```python
from build123d import *

# Parameters (mm, degrees)
SKETCH2_R                   = 8.255
BOSS_EXTRUDE1_DEPTH         = 6.35
BOSS_EXTRUDE1_DEPTH_BACK    = 6.35
BOSS_EXTRUDE2_DEPTH         = 10.16
BOSS_EXTRUDE2_DEPTH_BACK    = 16.256
SKETCH4_W                   = 20.32
SKETCH4_H                   = 10.16
BOSS_EXTRUDE3_DEPTH         = 10.16
BOSS_EXTRUDE3_DEPTH_BACK    = 16.51
SKETCH5_W                   = 20.32
SKETCH5_H                   = 10.16
CUT_EXTRUDE1_DEPTH          = 372.505050517
CUT_EXTRUDE2_DEPTH          = 370.547039673
CUT_EXTRUDE3_START          = -16.256
CUT_EXTRUDE3_DEPTH          = 16.256
CUT_EXTRUDE4_DEPTH          = 16.51
E_0_25_DIAMETER_HOLE1_D     = 6.35
E_0_25_DIAMETER_HOLE1_DEPTH = 19.05
E_0_25_DIAMETER_HOLE1_TIP   = 1.907732465
CUT_EXTRUDE5_DEPTH          = 367.61301524
CUT_EXTRUDE5_DEPTH_BACK     = 367.61301524
SKETCH13_R                  = 3.175


with BuildPart() as part:
    # Sweep1: sweep along a path in Sketch1
    with BuildLine(Plane(origin=(0, 0, 0), x_dir=(1, 0, 0), z_dir=(0, 1, 0))) as sweep1_path:
        Line((-307.263447944, -157.854259231), (0, 0))
        Line((0, 0), (-307.263447944, 172.345740769))
    # Sketch2 → Sweep1 (sweep)
    with BuildSketch(Plane(origin=(-307.263447944, 0, 157.854259231), x_dir=(-0.45696578054298637, 0, -0.8894842749665333), z_dir=(0.8894842749665333, 0, -0.45696578054298637))):
        Circle(SKETCH2_R)
    sweep(path=sweep1_path.line, transition=Transition.RIGHT)

    # Sketch3 → Boss-Extrude1 (add, two sides: drawn at the far end of the back side and taken through both)
    with BuildSketch(Plane.XY.offset(-BOSS_EXTRUDE1_DEPTH_BACK)):
        Polygon((33.931753368, 10.795), (11.09345, 10.795), (11.09345, -10.795), (33.931753368, -10.795), (33.931753368, -7.62), (14.26845, -7.62), (14.26845, 7.62), (33.931753368, 7.62), align=None)
    extrude(amount=BOSS_EXTRUDE1_DEPTH + BOSS_EXTRUDE1_DEPTH_BACK)

    # Sketch4 → Boss-Extrude2 (add, two sides: drawn at the far end of the back side and taken through both)
    with BuildSketch(Plane(origin=(-307.263447944, 0, 157.854259231), x_dir=(0.45696578054298637, 0, 0.8894842749665333), z_dir=(-0.8894842749665333, 0, 0.45696578054298637)).offset(-BOSS_EXTRUDE2_DEPTH_BACK)):
        Rectangle(SKETCH4_W, SKETCH4_H)
    extrude(amount=BOSS_EXTRUDE2_DEPTH + BOSS_EXTRUDE2_DEPTH_BACK)

    # Sketch5 → Boss-Extrude3 (add, two sides: drawn at the far end of the back side and taken through both)
    with BuildSketch(Plane(origin=(-307.263447944, 0, -172.345740769), x_dir=(-0.4892044257112748, 0, 0.8721691520940774), z_dir=(-0.8721691520940774, 0, -0.4892044257112748)).offset(-BOSS_EXTRUDE3_DEPTH_BACK)):
        Rectangle(SKETCH5_W, SKETCH5_H)
    extrude(amount=BOSS_EXTRUDE3_DEPTH + BOSS_EXTRUDE3_DEPTH_BACK)

    # Sketch6 → Cut-Extrude1 (cut, through all)
    with BuildSketch(Plane(origin=(0, 5.08, 0), x_dir=(1, 0, 0), z_dir=(0, 1, 0))):
        with BuildLine():
            Line((-312.23376491, 163.484502184), (-321.095003495, 168.454819149))
            Line((-321.095003495, 168.454819149), (-316.12468653, 177.316057734))
            ThreePointArc((-316.12468653, 177.316057734), (-317.043834669, 169.594443707), (-312.23376491, 163.484502184))
        make_face()
    cut_extrude1 = extrude(amount=-CUT_EXTRUDE1_DEPTH, mode=Mode.SUBTRACT)

    # Mirror1: Cut-Extrude1 across plane
    add(cut_extrude1.mirror(Plane(origin=(0, 0, 0), x_dir=(0.8721691520940776, 0, 0.48920442571127426), z_dir=(-0.4892044257112748, 0, 0.8721691520940775))), mode=Mode.SUBTRACT)

    # Sketch7 → Cut-Extrude2 (cut, through all)
    with BuildSketch(Plane(origin=(0, 5.08, 0), x_dir=(1, 0, 0), z_dir=(0, 1, 0))):
        with BuildLine():
            Line((-302.620675614, -166.891419464), (-311.657835848, -171.534191795))
            Line((-311.657835848, -171.534191795), (-316.300608178, -162.497031561))
            ThreePointArc((-316.300608178, -162.497031561), (-310.37074943, -167.527432313), (-302.620675614, -166.891419464))
        make_face()
    cut_extrude2 = extrude(amount=-CUT_EXTRUDE2_DEPTH, mode=Mode.SUBTRACT)

    # Mirror2: Cut-Extrude2 across plane
    add(cut_extrude2.mirror(Plane(origin=(0, 0, 0), x_dir=(-0.8894842749665333, 0, 0.45696578054298614), z_dir=(0.45696578054298637, 0, 0.8894842749665333))), mode=Mode.SUBTRACT)

    # Sketch8 → Cut-Extrude3 (cut)
    with BuildSketch(Plane(origin=(-307.263447944, 0, 157.854259231), x_dir=(0.45696578054298637, 0, 0.8894842749665333), z_dir=(-0.8894842749665333, 0, 0.45696578054298637)).offset(CUT_EXTRUDE3_START)):
        with BuildLine():
            Line((6.506813736, -5.08), (-6.506813736, -5.08))
            ThreePointArc((-6.506813736, -5.08), (0, -8.255), (6.506813736, -5.08))
        make_face()
        with BuildLine():
            Line((-6.506813736, 5.08), (6.506813736, 5.08))
            ThreePointArc((6.506813736, 5.08), (0, 8.255), (-6.506813736, 5.08))
        make_face()
    extrude(amount=CUT_EXTRUDE3_DEPTH, mode=Mode.SUBTRACT)

    # Sketch9 → Cut-Extrude4 (cut)
    with BuildSketch(Plane(origin=(-307.263447944, 0, -172.345740769), x_dir=(-0.4892044257112748, 0, 0.8721691520940774), z_dir=(-0.8721691520940774, 0, -0.4892044257112748))):
        with BuildLine():
            Line((6.506813736, -5.08), (-6.506813736, -5.08))
            ThreePointArc((-6.506813736, -5.08), (0, -8.255), (6.506813736, -5.08))
        make_face()
        with BuildLine():
            Line((-6.506813736, 5.08), (6.506813736, 5.08))
            ThreePointArc((6.506813736, 5.08), (0, 8.255), (-6.506813736, 5.08))
        make_face()
    extrude(amount=-CUT_EXTRUDE4_DEPTH, mode=Mode.SUBTRACT)

    # E (0.25) Diameter Hole1
    with Locations(Plane(origin=(-307.263447944, 5.08, -172.345740769), x_dir=(0, 0, 1), z_dir=(0, 1, 0))):
        with Locations((0, 0), (330.2, 0)):
            Hole(E_0_25_DIAMETER_HOLE1_D / 2, depth=E_0_25_DIAMETER_HOLE1_DEPTH)
            with Locations((0, 0, -(E_0_25_DIAMETER_HOLE1_DEPTH + E_0_25_DIAMETER_HOLE1_TIP / 2))):  # 118° drill point
                Cone(0, E_0_25_DIAMETER_HOLE1_D / 2, E_0_25_DIAMETER_HOLE1_TIP, mode=Mode.SUBTRACT)

    # Sketch13 → Cut-Extrude5 (cut, two sides: drawn at the far end of the back side and taken through both)
    with BuildSketch(Plane(origin=(0, -7.62, 0), x_dir=(1, 0, 0), z_dir=(0, 1, 0)).offset(-CUT_EXTRUDE5_DEPTH_BACK)):
        with Locations(Location((24.100101684, 0, 0), (0, 0, 180))):
            Circle(SKETCH13_R)
    extrude(amount=CUT_EXTRUDE5_DEPTH + CUT_EXTRUDE5_DEPTH_BACK, mode=Mode.SUBTRACT)


solid = part.part
```
The listing builds one solid part. Answer for the finished solid, in the listing's coordinates (mm). A direction names the side the tool comes from. Give positions to 0.01 mm unless a question says otherwise; leave off trailing zeros. One line per item, written item: value.
1) Flat-ended cylindrical pins translate along their axes: P1, Ø1.5, axis at y = 2, z = -36, coming from the +X side; P2, Ø4, axis at y = -3.5, z = 1.5, coming from the -X side; P3, Ø1.5, axis at y = 1, z = 22, coming from the -X side; P4, Ø10, axis at x = 22, z = 0, coming from the +Y side (3 decimals). Find the tip coordinate at first contact, or state that the pin passes through.
Reported:
P1: stops at x = -46.42
P2: stops at x = -23.56
P3: stops at x = -62.23
P4: stops at y = 10.795
2) A tool of negligible diameter and unlimited length cuts with its end or side. For faces 4 (the flat face through (-304, 5.08, -171)), 5 (the flat face through (14.268, 0, -2)), 6 (the flat face through (14, 0, 6.35)), 7 (the flat face through (-304.575, -0.071, 145.051)), 8 (the flat face through (-304, 5.08, 156)), from which of +Z, -Z, +X, -X, +Y, -Y can it reach the whole face along a straight path? Write none if from no direction.
Reported:
face 4: -Z, -X, +Y
face 5: +X
face 6: +Z, +X, +Y, -Y
face 7: -X, +Y, -Y
face 8: +Z, -X, +Y
3) Determine the mould class of faces 1 (the flat face through (11.093, 3, -3)), 2 (the flat face through (-304, -5.08, 156)), 3 (the flat face through (-304.93, -0.07, -159.39)) for opening direction X: pulls with the +X half, pulls with the -X half, needs draft (parallel to the pull), parting line crosses it, or undercut.
Reported:
face 1: undercut
face 2: needs draft
face 3: pulls with the -X half
4) Find the intervals of material crossed by line 1 (X direction, y = -9.5, z = 0); line 2 (Z direction, x = -147.5, y = -3.5); line 3 (Z direction, x = -274, y = 3.25), in increasing order.
Reported:
line 1: x = 11.09 to 20.93, 27.28 to 33.93
line 2: z = -91.31 to -74.16, 67.37 to 84.18
line 3: z = -162.39 to -144.99, 132.23 to 149.3
